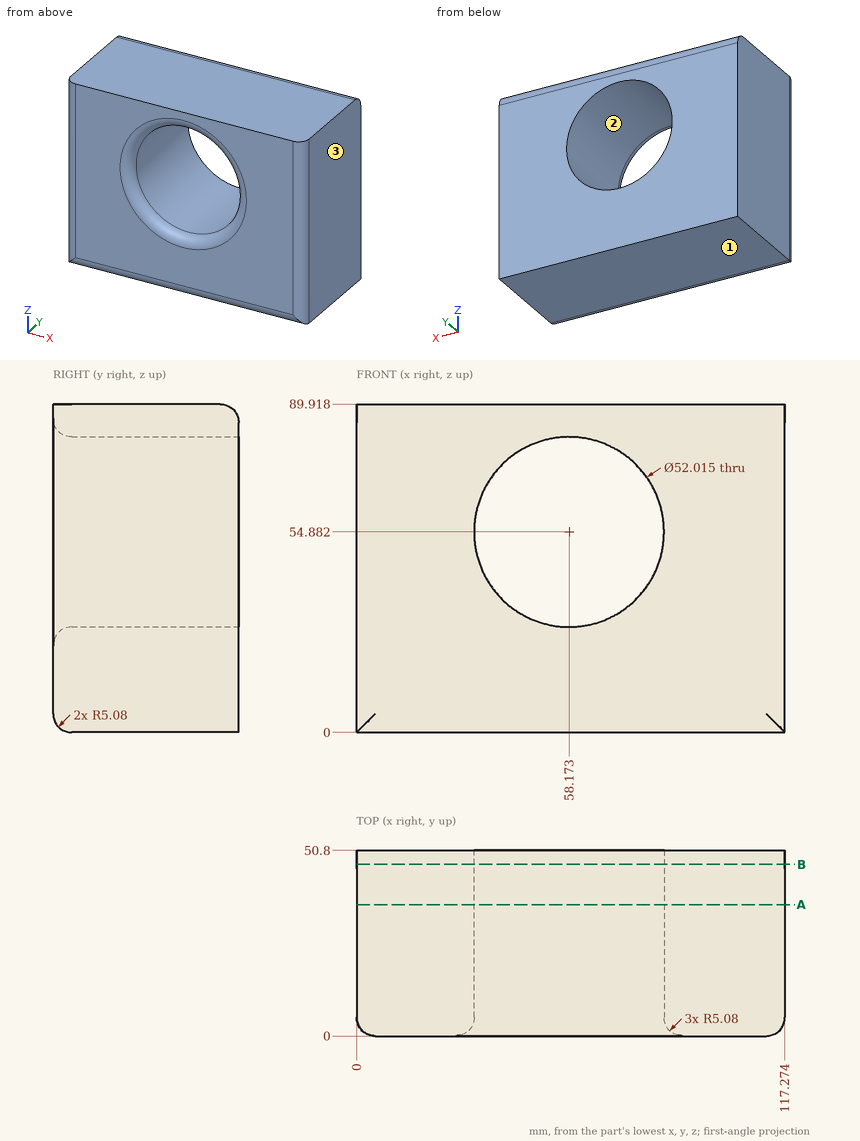
Design review of the part shown in the three views and the two pictorial views. Dimensions are in mm from the part's minimum x, y and z. Coordinates: 2 decimals unless noted, no trailing zeros. Order: outer loops, then holes, each group sorted by start corner. A loop starts at its lowest first (then second) coordinate and runs counter-clockwise, first axis right, second up. Notation, with made-up numbers: (51.25, -16) -> (72.25, -16) arc R24 cw to (72.25, 4) -> close; hole circle Ø6 at (28.5, 38.25). An arc over 180 degrees is marked (long way). Use one line per item in the form item = value. Start each with the question number.
(1) Insertion check: pin 1 (8 mm diameter, centred on x = 82.5, z = 58.5, fed in from -Y). The pin has a flat end and moves straight along its axis. Give the tip position at first contact, or say it passes through.
(2) Add section B-B on y = 47. State the section outline as (x, z) points (1 decimal), plus the area to 3 significant figures.
(3) For probe 1 along Z at (x, y) = (59, 16); probe 2 along Z at (x, y) = (45.5, 44); probe 3 along X at (y, z) = (44.5, 32) (1 decimal), list the stretches that pass through material, from the lowest coordinate up.
(4) Add section A-A on y = 36. State the section outline as (x, z) points (1 decimal).
(5) The part is to be moulded in two halves that separate along Z. For the marked faces 1, 2 and 3, say which applies: +Z half, -Z half, draft (parallel to the pull), parting line (faces both ways), or undercut.
Answer block:
q1.pin_1 = 0.65
q2.outline = (0, 0) -> (117.3, 0) -> (117.3, 89.8) -> (0, 89.8) -> close; hole circle Ø52 at (58.2, 54.9)
q2.area = 8,400 mm²
q3.probe_1 = 0 to 28.89, 80.88 to 89.92
q3.probe_2 = 0 to 32.17, 77.59 to 89.92
q3.probe_3 = 0 to 45.8, 70.5 to 117.3
q4.outline = (0, 0) -> (117.3, 0) -> (117.3, 89.9) -> (0, 89.9) -> close; hole circle Ø52 at (58.2, 54.9)
q5.face_1 = -Z half
q5.face_2 = undercut
q5.face_3 = draft
